```python
from build123d import *

# Parameters (mm, degrees)
BOSS_EXTRUDE1_DEPTH = 15.85
SKETCH2_R           = 2.45
BOSS_EXTRUDE2_DEPTH = 1.8
SKETCH3_W           = 12.85
SKETCH3_H           = 6.5
CUT_EXTRUDE1_DEPTH  = 2.05
SKETCH4_R           = 0.95
CUT_EXTRUDE2_DEPTH  = 1.5
SKETCH5_R           = 1.5
SKETCH5_R_2         = 0.7
BOSS_EXTRUDE3_DEPTH = 1.85
SKETCH6_R           = 2.45
SKETCH6_R_2         = 1.55
BOSS_EXTRUDE4_DEPTH = 1.8
FILLET1_R           = 0.5


with BuildPart() as part:
    # Sketch1 → Boss-Extrude1 (new body)
    with BuildSketch(Plane(origin=(0, 0, 0), x_dir=(0, 0, -1), z_dir=(1, 0, 0))):
        Polygon((0, 16), (0, 0), (9.6, 0), (9.6, 3.25), (1.55, 3.25), (1.55, 16), align=None)
    extrude(amount=-BOSS_EXTRUDE1_DEPTH)

    # Sketch2 → Boss-Extrude2 (add)
    with BuildSketch(Plane(origin=(0, 3.25, 0), x_dir=(1, 0, 0), z_dir=(0, 1, 0))):
        with Locations(Location((-11.8875, 5.575, 0), (0, 0, 270))):
            Circle(SKETCH2_R)
        with Locations(Location((-3.9625, 5.575, 0), (0, 0, 270))):
            Circle(SKETCH2_R)
    extrude(amount=BOSS_EXTRUDE2_DEPTH)

    # Sketch3 → Cut-Extrude1 (cut)
    with BuildSketch(Plane.XZ):
        with Locations((-7.925, -4.85)):
            Rectangle(SKETCH3_W, SKETCH3_H)
    extrude(amount=-CUT_EXTRUDE1_DEPTH, mode=Mode.SUBTRACT)

    # Sketch4 → Cut-Extrude2 (cut)
    with BuildSketch(Plane.XZ.offset(-2.05)):
        with Locations(Location((-11.8875, -5.575, 0), (0, 0, 270))):
            Circle(SKETCH4_R)
        with Locations(Location((-3.9625, -5.575, 0), (0, 0, 270))):
            Circle(SKETCH4_R)
    extrude(amount=-CUT_EXTRUDE2_DEPTH, mode=Mode.SUBTRACT)

    # Sketch5 → Boss-Extrude3 (add)
    with BuildSketch(Plane.XZ.offset(-2.05)):
        with Locations(Location((-7.925, -5.57, 0), (0, 0, 270))):
            Circle(SKETCH5_R)
        with Locations(Location((-7.925, -5.57, 0), (0, 0, 270))):
            Circle(SKETCH5_R_2, mode=Mode.SUBTRACT)
    extrude(amount=BOSS_EXTRUDE3_DEPTH)

    # Sketch6 → Boss-Extrude4 (add)
    # profile 1 of 4: a face of its own
    with BuildSketch(Plane.XY):
        with Locations((-11.8875, 12)):
            Circle(SKETCH6_R)
        with Locations(Location((-11.8875, 12, 0), (0, 0, 270))):
            Circle(SKETCH6_R_2, mode=Mode.SUBTRACT)
    # profile 2 of 4: a face of its own
    with BuildSketch(Plane.XY):
        with Locations((-3.9675, 12)):
            Circle(SKETCH6_R)
        with Locations(Location((-3.9675, 12, 0), (0, 0, 270))):
            Circle(SKETCH6_R_2, mode=Mode.SUBTRACT)
    # profile 3 of 4: a face of its own
    with BuildSketch(Plane.XY):
        with Locations((-3.9625, 4.000001563)):
            Circle(SKETCH6_R)
        with Locations(Location((-3.9625, 4.000001563, 0), (0, 0, 270))):
            Circle(SKETCH6_R_2, mode=Mode.SUBTRACT)
    # profile 4 of 4: a face of its own
    with BuildSketch(Plane.XY):
        with Locations((-11.8825, 4.000001563)):
            Circle(SKETCH6_R)
        with Locations(Location((-11.8825, 4.000001563, 0), (0, 0, 270))):
            Circle(SKETCH6_R_2, mode=Mode.SUBTRACT)
    extrude(amount=BOSS_EXTRUDE4_DEPTH)

    # Fillet1
    fillet1_edges = [part.edges().sort_by_distance(p)[0] for p in [
        (-15.85, 16, -0.775),
        (0, 16, -0.775),
    ]]
    fillet(fillet1_edges, radius=FILLET1_R)


solid = part.part
```
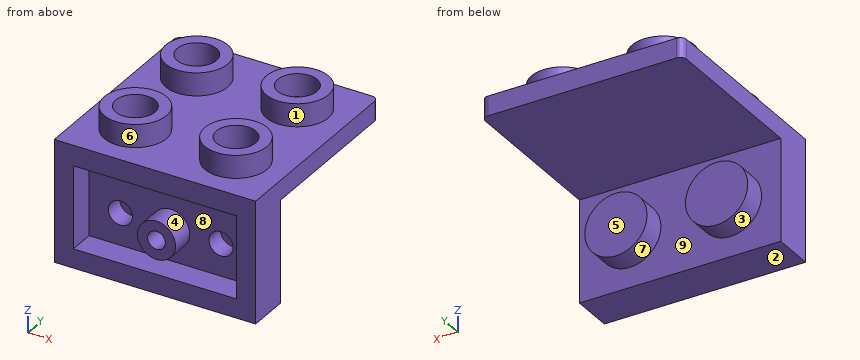
Work out the finished part from the listing and answer in its coordinate system (mm). Face numbers are marked on the shaded views. A direction names the side the tool comes from. Coordinates: 2 decimals unless noted, no trailing zeros. Loops run counter-clockwise (first coordinate to the right, second up) from the corner with the lowest first, then second, coordinate; pieces in that order, holes last. Notation, with made-up numbers: M -9.5,69.5 L 25.5,69.5 A6 cw 25.5,74.5 Z; hole C 31,-13 d7. An arc over 180 degrees is marked long. Use CSV: the item, a comma, the result in double quotes. Start each with the question number.
(1) Find section A-A, the plane z = 1. Give the vertices of the cut face in (x, y), then the cut area to 3 significant figures.
(2) Consider line 1 (X direction, y = 12.25, z = 1); line 2 (X direction, y = 1.5, z = -2); line 3 (Y direction, x = -15, z = -2). Determine where each line is inside the solid, lowest interval first.
(3) Given pin 1 Ø2.5 at (x, y) = (-3.5, 4) entering from +Z; pin 2 Ø0.9 at (x, y) = (-12.5, 4) entering from +Z; pin 3 Ø1.7 at (x, z) = (-11.89, -5.58) entering from +Y; pin 4 Ø0.9 at (x, z) = (-4.5, -6) entering from -Y, each flat-ended and moving along its own axis, determine where each tip first touches the part or whether it passes through.
(4) Find section B-B, the plane y = 12. Give the vertices of the cut face in (x, z), then the cut area to 3 significant figures.
(5) For a pull along Y with two mould halves and no side action, classify the marked faces 6, 7, 8 and 9 as +Y half, -Y half, draft (parallel to the pull), parting line (faces both ways), or undercut.
(6) Find section C-C, the plane y = 4.5. State how many separate pieces and enclosed holes the cut face has, then the cut area to 3 significant figures.
(7) For the marked faces 1, 2, 3, 4 and 5, determine the directions among +Z, -Z, +X, -X, +Y, -Y from which every point of the face is accessible in a straight line to the end or side of a thin tool.
(8) Find section D-D, the plane x = -9. Give the vertices of the cut face in (y, z).
Recorded:
1,outline,"C -11.89,12 d4.9; C -11.88,4 d4.9; C -3.97,12 d4.9; C -3.96,4 d4.9; hole C -11.89,12 d3.1; hole C -11.88,4 d3.1; hole C -3.97,12 d3.1; hole C -3.96,4 d3.1"
1,area,"45.2 mm^2"
2,line 1,"x = -14.32 to -13.42, -10.36 to -9.45, -6.4 to -5.5, -2.44 to -1.53"
2,line 2,"x = -15.85 to -14.35, -1.5 to 0"
2,line 3,"y = 0 to 3.25"
3,pin 1,"stops at z = 1.8"
3,pin 2,"stops at z = 0"
3,pin 3,"stops at y = 5.05"
3,pin 4,"stops at y = 2.05"
4,outline,"M -15.85,-1.55 L 0,-1.55 L 0,0 L -1.52,0 L -1.52,1.8 L -2.42,1.8 L -2.42,0 L -5.52,0 L -5.52,1.8 L -6.42,1.8 L -6.42,0 L -9.44,0 L -9.44,1.8 L -10.34,1.8 L -10.34,0 L -13.44,0 L -13.44,1.8 L -14.34,1.8 L -14.34,0 L -15.85,0 Z"
4,area,"31.0 mm^2"
5,face 6,"undercut"
5,face 7,"draft"
5,face 8,"-Y half"
5,face 9,"+Y half"
6,separate pieces,"3"
6,enclosed holes,"0"
6,area,"69.0 mm^2"
7,face 1,"+Z"
7,face 2,"-Z, +X, -X, +Y, -Y"
7,face 3,"+Y"
7,face 4,"-Y"
7,face 5,"-Z, +X, -X, +Y"
8,outline,"M 0,-9.6 L 3.25,-9.6 L 3.25,-1.55 L 16,-1.55 L 16,0 L 0,0 L 0,-1.6 L 2.05,-1.6 L 2.05,-4.52 L 0.2,-4.52 L 0.2,-6.62 L 2.05,-6.62 L 2.05,-8.1 L 0,-8.1 Z"
